from build123d import *

# Parameters (mm, degrees)
SKETCH_1_R          = 13.5
SKETCH_1_R_2        = 1.95
EXTRUDE_1_DEPTH     = 3
SKETCH_2_R          = 1.45
CUT_EXTRUDE_1_DEPTH = 10
FILLET_1_R          = 3
CUT_EXTRUDE_2_DEPTH = 52.529117982
FILLET_2_R          = 1.5


with BuildPart() as part:
    # 草图1 → 凸台-拉伸1 (new body)
    with BuildSketch(Plane.XY):
        with BuildLine():
            Line((-22, 0), (-22, -46.5))
            Line((-22, -46.5), (22, -46.5))
            Line((22, -46.5), (22, 0))
            ThreePointArc((22, 0), (0, 22), (-22, 0))
        make_face()
        Circle(SKETCH_1_R, mode=Mode.SUBTRACT)
        with Locations((0, 17.5)):
            Circle(SKETCH_1_R_2, mode=Mode.SUBTRACT)
        with Locations((17.5, 0)):
            Circle(SKETCH_1_R_2, mode=Mode.SUBTRACT)
        with Locations((-17.5, 0)):
            Circle(SKETCH_1_R_2, mode=Mode.SUBTRACT)
        with Locations((0, -17.5)):
            Circle(SKETCH_1_R_2, mode=Mode.SUBTRACT)
    extrude(amount=EXTRUDE_1_DEPTH)

    # 草图2 → 切除-拉伸1 (cut)
    with BuildSketch(Plane.XY.offset(3)):
        with Locations((0, -41.5)):
            Circle(SKETCH_2_R)
        with Locations((17, -41.5)):
            Circle(SKETCH_2_R)
        with Locations((-17, -41.5)):
            Circle(SKETCH_2_R)
        with Locations((-17, -29.5)):
            Circle(SKETCH_2_R)
        with Locations((17, -29.5)):
            Circle(SKETCH_2_R)
    extrude(amount=-CUT_EXTRUDE_1_DEPTH, mode=Mode.SUBTRACT)

    # 圆角1
    fillet_1_edges = [part.edges().sort_by_distance(p)[0] for p in [
        (22, -46.5, 1.5),
        (-22, -46.5, 1.5),
    ]]
    fillet(fillet_1_edges, radius=FILLET_1_R)

    # 草图3 → 切除-拉伸2 (cut, through all)
    with BuildSketch(Plane.XY.offset(3)):
        Polygon((17.752585541, -7.827536111), (10.726827306, -43.019057271), (2.50919937, -39.255258217), (2.50919937, -22.502580513), align=None)
        Polygon((-17.062555714, -8.580295922), (-2.571929354, -22.321407125), (-2.571929354, -39.255258217), (-11.667777069, -42.266297461), align=None)
    extrude(amount=-CUT_EXTRUDE_2_DEPTH, mode=Mode.SUBTRACT)

    # 圆角2
    fillet_2_edges = [part.edges().sort_by_distance(p)[0] for p in [
        (2.50919937, -22.502580513, 1.5),
        (17.752585541, -7.827536111, 1.5),
        (10.726827306, -43.019057271, 1.5),
        (2.50919937, -39.255258217, 1.5),
        (-11.667777069, -42.266297461, 1.5),
        (-17.062555714, -8.580295922, 1.5),
        (-2.571929354, -22.321407125, 1.5),
        (-2.571929354, -39.255258217, 1.5),
    ]]
    fillet(fillet_2_edges, radius=FILLET_2_R)


solid = part.part
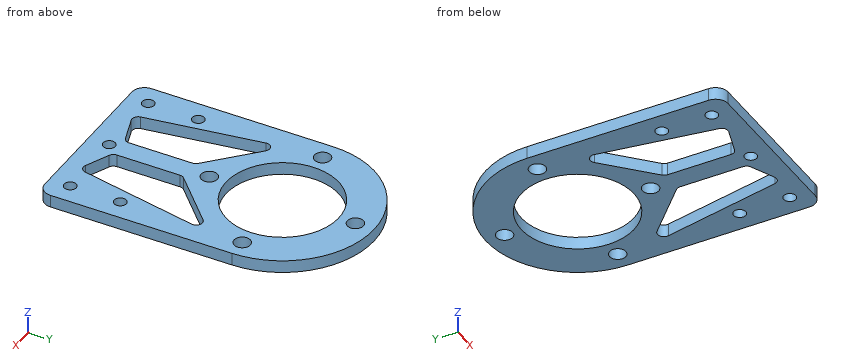
The listing builds one solid part. Answer for the finished solid, in the listing's coordinates (mm). Coordinates: 2 decimals unless noted, no trailing zeros. Write each loop counter-clockwise with the first axis right and the second up, starting at its lowest first coordinate (ties: lowest second). Pieces come first, ordered by that corner, then holes. Notation, with made-up numbers: (35, -37.5) - (61, -37.5) arc R10 ccw to (61, -24.5) - close; hole circle Ø11 at (78.5, -9.75). An arc over 180 degrees is marked (long way). Return JSON: item names as keys, results as strings.
1. The part is cut by section A-A on x = 0. Determine the outline of the cut face in (y, z), then the cut area to 3 significant figures.
Final values:
{"outline": "(-46.5, 0) - (-42.95, 0) - (-42.95, 3) - (-46.5, 3) - close; (-40.05, 0) - (-19.45, 0) - (-19.45, 3) - (-40.05, 3) - close; (-15.55, 0) - (-13.5, 0) - (-13.5, 3) - (-15.55, 3) - close; (13.5, 0) - (15.55, 0) - (15.55, 3) - (13.5, 3) - close; (19.45, 0) - (22, 0) - (22, 3) - (19.45, 3) - close", "area": "92.4 mm^2"}
2. The part is cut by section D-D on x = -5. Determine the outline of the cut face in (y, z), then the cut area to 3 significant figures.
Final values:
{"outline": "(-46.5, 0) - (-40.06, 0) - (-40.06, 3) - (-46.5, 3) - close; (-20.02, 0) - (-12.54, 0) - (-12.54, 3) - (-20.02, 3) - close; (12.54, 0) - (21.42, 0) - (21.42, 3) - (12.54, 3) - close", "area": "68.4 mm^2"}
3. Consider line 1 along Y through (x, z) = (0, 2); line 2 along X through (y, z) = (-1.5, 2.7); line 3 along Y through (x, z) = (-17, 0.75). Determine where each line is inside the solid, lowest interval first.
Final values:
{"line 1": "-46.5 to -42.95, -40.05 to -19.45, -15.55 to -13.5, 13.5 to 15.55, 19.45 to 22", "line 2": "-22 to -18.75, -16.25 to -13.42, 13.42 to 16.25, 18.75 to 22", "line 3": "-46.5 to -42.95, -40.05 to -30.95, -28.05 to -1.88, 1.88 to 13.96"}
4. This flat-tipped pin is pushed along its axis until it touches: pin 1 Ø1 at (x, z) = (-3, 2.5) entering from +Y. Where does it stop, or does it pass through?
Final values:
{"pin 1": "y = 21.86"}
5. The part is cut by section C-C on y = 17.5. Determine the outline of the cut face in (x, z), then the cut area to 3 significant figures.
Final values:
{"outline": "(-13.33, 0) - (-1.95, 0) - (-1.95, 3) - (-13.33, 3) - close; (1.95, 0) - (13.33, 0) - (13.33, 3) - (1.95, 3) - close", "area": "68.3 mm^2"}
6. The part is cut by section B-B on z = 0.85. Count the separate pieces of the cut face and the enclosed holes in it, then the cut area to 3 significant figures.
Final values:
{"separate pieces": "1", "enclosed holes": "12", "area": "1,590 mm^2"}
